```python
from build123d import *

# Parameters (mm, degrees)
F3_DEPTH = 10


with BuildPart() as f3:
    # F2 (on Front) → F3 (new body)
    with BuildSketch(Plane.XZ):
        with BuildLine():
            ThreePointArc((400, -100), (447.127307, -97.214069), (493.598148, -88.895084))
            ThreePointArc((493.598148, -88.895084), (505.426816, -61.311377), (511.379193, -31.894588))
            Line((511.379193, -31.894588), (510.98747, 0))
            Line((510.98747, 0), (500.98747, 0))
            Line((500.98747, 0), (501.038948, -4.191425))
            ThreePointArc((501.038948, -4.191425), (493.129496, -37.67403), (474.561698, -66.637476))
            ThreePointArc((474.561698, -66.637476), (440.842701, -91.279098), (400, -100))
        make_face()
        with BuildLine():
            Line((5.98747, 22.610795), (5.98747, -29.484774))
            ThreePointArc((5.98747, -29.484774), (192.466811, -126.522127), (400, -160))
            ThreePointArc((400, -160), (454.252189, -134.258366), (493.598148, -88.895084))
            ThreePointArc((493.598148, -88.895084), (447.127307, -97.214069), (400, -100))
            ThreePointArc((400, -100), (142.687028, -6.251587), (5.98747, 231.049827))
            Line((5.98747, 231.049827), (5.98747, 22.610795))
        make_face()
    extrude(amount=F3_DEPTH)


solid = f3.part
```
Model file for the job. Use its own axes, mm. A direction names the side the tool comes from. Round coordinates to 2 decimals unless told otherwise and drop trailing zeros. Write each loop counter-clockwise with the first axis right and the second up, starting at its lowest first coordinate (ties: lowest second). Pieces come first, ordered by that corner, then holes. Notation, with made-up numbers: (61, 34.25) -> (93, 34.25) arc R14 ccw to (93, 42.25) -> close; hole circle Ø5 at (-37, 69.25). An arc over 180 degrees is marked (long way). Answer as CSV lines item,"result".
1. Slice it at B-B, the plane x = 197.5. List the corners of the cut face in (y, z).
Resolved:
outline,"(-10, -128.17) -> (0, -128.17) -> (0, -44.95) -> (-10, -44.95) -> close"
2. Slice it at A-A, the plane y = -5.25. List the corners of the cut face in (x, z).
Resolved:
outline,"(5.99, -29.48) arc R660 ccw to (400, -160) arc R146.34 ccw to (493.6, -88.9) arc R146.34 ccw to (511.38, -31.89) -> (510.99, 0) -> (500.99, 0) -> (501.04, -4.19) arc R102.24 cw to (474.56, -66.64) arc R100 cw to (400, -100) arc R400 cw to (5.99, 231.05) -> close"
3. Slice it at C-C, the plane z = 195.5. List the corners of the cut face in (x, y), plus the area to 3 significant figures.
Resolved:
outline,"(5.99, -10) -> (13.89, -10) -> (13.89, 0) -> (5.99, 0) -> close"
area,"79.0 mm²"
4. Pin check, flat tips, straight feed: pin 1 Ø3 at (x, y) = (506.5, -4.5) entering from +Z; pin 2 Ø3 at (x, y) = (204, -3.5) entering from +Z; pin 3 Ø5 at (y, z) = (-7, -103.5) entering from -X. Stop position of each tip, or through.
Resolved:
pin 1,"z = 0"
pin 2,"z = -47.84"
pin 3,"x = 127.24"
5. Drill centre lines: line 1 (Z direction, x = 42, y = -0.25); line 2 (X direction, y = -2, z = 48.5); line 3 (X direction, y = -5.75, z = 200). Where is each one in solid material? Low to high.
Resolved:
line 1,"-54.47 to 121.57"
line 2,"5.99 to 88.96"
line 3,"5.99 to 12.7"
6. Mould opens along X. For faces 4 (the face through (493.317, -4.93, -37.228)), 5 (the face through (5.987, -5, 103)), 6 (the face through (182.6, -10, -36)) say: +X half, -X half, draft (parallel to the pull), parting line (faces both ways), or undercut.
Resolved:
face 4,"undercut"
face 5,"-X half"
face 6,"draft"
7. Tool access for faces 1 (the face through (145.695, -4.93, -8.754)), 2 (the face through (189.7, -4.9, -125.6)), 3 (the face through (506, -5, 0)): list every direction of +Z, -Z, +X, -X, +Y, -Y with a clear straight run to the whole face (end or side of a thin tool).
Resolved:
face 1,"+Z, +Y, -Y"
face 2,"-Z, -X, +Y, -Y"
face 3,"+Z, +X, +Y, -Y"
